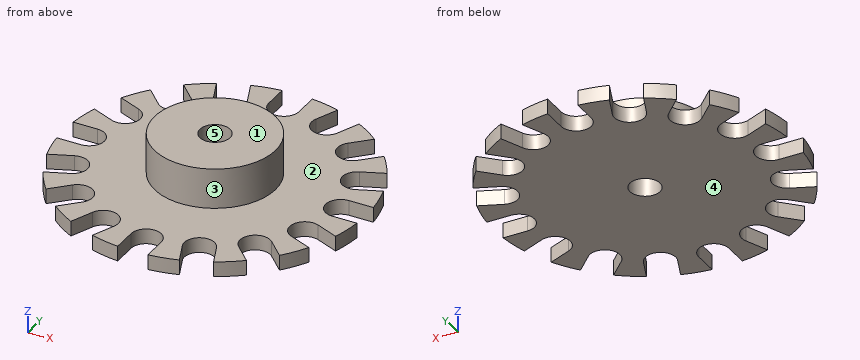
```python
from build123d import *

# Parameters (mm, degrees)
SKETCH1_R           = 15
SKETCH1_R_2         = 1.5
BOSS_EXTRUDE1_DEPTH = 1.5
SKETCH2_R           = 6
SKETCH2_R_2         = 1.5
BOSS_EXTRUDE2_DEPTH = 4
SKETCH3_R           = 1.5
CUT_EXTRUDE3_DEPTH  = 22.587033145


with BuildPart() as part:
    # Sketch1 → Boss-Extrude1 (new body)
    with BuildSketch(Plane.XY):
        Circle(SKETCH1_R)
        Circle(SKETCH1_R_2, mode=Mode.SUBTRACT)
    extrude(amount=BOSS_EXTRUDE1_DEPTH)

    # Sketch2 → Boss-Extrude2 (add)
    with BuildSketch(Plane.XY.offset(1.5)):
        Circle(SKETCH2_R)
        Circle(SKETCH2_R_2, mode=Mode.SUBTRACT)
    extrude(amount=BOSS_EXTRUDE2_DEPTH)

    # Sketch3 → Cut-Extrude3 (cut, through all)
    with BuildSketch(Plane.XY.offset(1.5)):
        with BuildLine():
            ThreePointArc((-1.5, 12.5), (0, 14), (1.5, 12.5))
            Line((1.5, 12.5), (1.5, 14.924811557))
            ThreePointArc((1.5, 14.924811557), (0, 15), (-1.5, 14.924811557))
            Line((-1.5, 14.924811557), (-1.5, 12.5))
        make_face()
        with Locations((0, 12.5)):
            Circle(SKETCH3_R)
        with Locations((4.783542905, 11.548494156)):
            Circle(SKETCH3_R)
        with BuildLine():
            ThreePointArc((7.097297413, 13.214702775), (5.740251485, 13.858192988), (4.325658815, 14.362753072))
            Line((4.325658815, 14.362753072), (3.397723606, 12.122519305))
            ThreePointArc((3.397723606, 12.122519305), (5.076178388, 13.019672077), (6.283542905, 11.548494156))
            ThreePointArc((6.283542905, 11.548494156), (6.254720825, 11.255858673), (6.169362203, 10.974469008))
            Line((6.169362203, 10.974469008), (7.097297413, 13.214702775))
        make_face()
        with Locations((8.838834765, 8.838834765)):
            Circle(SKETCH3_R)
        with BuildLine():
            ThreePointArc((11.614095631, 9.492775288), (10.606601718, 10.606601718), (9.492775288, 11.614095631))
            Line((9.492775288, 11.614095631), (7.778174593, 9.899494937))
            ThreePointArc((7.778174593, 9.899494937), (9.412859913, 10.224654064), (10.338834765, 8.838834765))
            ThreePointArc((10.338834765, 8.838834765), (10.224654064, 8.264809616), (9.899494937, 7.778174593))
            Line((9.899494937, 7.778174593), (11.614095631, 9.492775288))
        make_face()
        with Locations((11.548494156, 4.783542905)):
            Circle(SKETCH3_R)
        with BuildLine():
            ThreePointArc((14.362753072, 4.325658815), (13.858192988, 5.740251485), (13.214702775, 7.097297413))
            Line((13.214702775, 7.097297413), (10.974469008, 6.169362203))
            ThreePointArc((10.974469008, 6.169362203), (12.381849506, 6.030747323), (13.048494156, 4.783542905))
            ThreePointArc((13.048494156, 4.783542905), (12.795698575, 3.950187555), (12.122519305, 3.397723606))
            Line((12.122519305, 3.397723606), (14.362753072, 4.325658815))
        make_face()
        with Locations((12.5, 0)):
            Circle(SKETCH3_R)
        with BuildLine():
            ThreePointArc((15, 0), (14.981191097, 0.750941626), (14.924811557, 1.5))
            Line((14.924811557, 1.5), (12.5, 1.5))
            ThreePointArc((12.5, 1.5), (13.560660172, 1.060660172), (14, 0))
            ThreePointArc((14, 0), (13.560660172, -1.060660172), (12.5, -1.5))
            Line((12.5, -1.5), (14.924811557, -1.5))
            ThreePointArc((14.924811557, -1.5), (14.981191097, -0.750941626), (15, 0))
        make_face()
        with Locations((11.548494156, -4.783542905)):
            Circle(SKETCH3_R)
        with BuildLine():
            ThreePointArc((13.214702775, -7.097297413), (13.858192988, -5.740251485), (14.362753072, -4.325658815))
            Line((14.362753072, -4.325658815), (12.122519305, -3.397723606))
            ThreePointArc((12.122519305, -3.397723606), (12.795698575, -3.950187555), (13.048494156, -4.783542905))
            ThreePointArc((13.048494156, -4.783542905), (12.381849506, -6.030747323), (10.974469008, -6.169362203))
            Line((10.974469008, -6.169362203), (13.214702775, -7.097297413))
        make_face()
        with BuildLine():
            ThreePointArc((9.492775288, -11.614095631), (10.606601718, -10.606601718), (11.614095631, -9.492775288))
            Line((11.614095631, -9.492775288), (9.899494937, -7.778174593))
            ThreePointArc((9.899494937, -7.778174593), (10.224654064, -8.264809616), (10.338834765, -8.838834765))
            ThreePointArc((10.338834765, -8.838834765), (9.412859913, -10.224654064), (7.778174593, -9.899494937))
            Line((7.778174593, -9.899494937), (9.492775288, -11.614095631))
        make_face()
        with Locations((8.838834765, -8.838834765)):
            Circle(SKETCH3_R)
        with Locations((4.783542905, -11.548494156)):
            Circle(SKETCH3_R)
        with BuildLine():
            ThreePointArc((4.325658815, -14.362753072), (5.740251485, -13.858192988), (7.097297413, -13.214702775))
            Line((7.097297413, -13.214702775), (6.169362203, -10.974469008))
            ThreePointArc((6.169362203, -10.974469008), (6.254720825, -11.255858673), (6.283542905, -11.548494156))
            ThreePointArc((6.283542905, -11.548494156), (5.076178388, -13.019672077), (3.397723606, -12.122519305))
            Line((3.397723606, -12.122519305), (4.325658815, -14.362753072))
        make_face()
        with BuildLine():
            ThreePointArc((-1.5, -14.924811557), (0, -15), (1.5, -14.924811557))
            Line((1.5, -14.924811557), (1.5, -12.5))
            ThreePointArc((1.5, -12.5), (0, -14), (-1.5, -12.5))
            Line((-1.5, -12.5), (-1.5, -14.924811557))
        make_face()
        with Locations((0, -12.5)):
            Circle(SKETCH3_R)
        with Locations((-4.783542905, -11.548494156)):
            Circle(SKETCH3_R)
        with BuildLine():
            Line((-6.169362203, -10.974469008), (-7.097297413, -13.214702775))
            ThreePointArc((-7.097297413, -13.214702775), (-5.740251485, -13.858192988), (-4.325658815, -14.362753072))
            Line((-4.325658815, -14.362753072), (-3.397723606, -12.122519305))
            ThreePointArc((-3.397723606, -12.122519305), (-5.357568053, -12.934313455), (-6.169362203, -10.974469008))
        make_face()
        with BuildLine():
            Line((-9.899494937, -7.778174593), (-11.614095631, -9.492775288))
            ThreePointArc((-11.614095631, -9.492775288), (-10.606601718, -10.606601718), (-9.492775288, -11.614095631))
            Line((-9.492775288, -11.614095631), (-7.778174593, -9.899494937))
            ThreePointArc((-7.778174593, -9.899494937), (-9.899494937, -9.899494937), (-9.899494937, -7.778174593))
        make_face()
        with Locations((-8.838834765, -8.838834765)):
            Circle(SKETCH3_R)
        with BuildLine():
            Line((-12.122519305, -3.397723606), (-14.362753072, -4.325658815))
            ThreePointArc((-14.362753072, -4.325658815), (-13.858192988, -5.740251485), (-13.214702775, -7.097297413))
            Line((-13.214702775, -7.097297413), (-10.974469008, -6.169362203))
            ThreePointArc((-10.974469008, -6.169362203), (-12.934313455, -5.357568053), (-12.122519305, -3.397723606))
        make_face()
        with Locations((-11.548494156, -4.783542905)):
            Circle(SKETCH3_R)
        with BuildLine():
            Line((-12.5, 1.5), (-14.924811557, 1.5))
            ThreePointArc((-14.924811557, 1.5), (-15, 0), (-14.924811557, -1.5))
            Line((-14.924811557, -1.5), (-12.5, -1.5))
            ThreePointArc((-12.5, -1.5), (-14, 0), (-12.5, 1.5))
        make_face()
        with Locations((-12.5, 0)):
            Circle(SKETCH3_R)
        with Locations((-11.548494156, 4.783542905)):
            Circle(SKETCH3_R)
        with BuildLine():
            Line((-10.974469008, 6.169362203), (-13.214702775, 7.097297413))
            ThreePointArc((-13.214702775, 7.097297413), (-13.858192988, 5.740251485), (-14.362753072, 4.325658815))
            Line((-14.362753072, 4.325658815), (-12.122519305, 3.397723606))
            ThreePointArc((-12.122519305, 3.397723606), (-12.934313455, 5.357568053), (-10.974469008, 6.169362203))
        make_face()
        with Locations((-8.838834765, 8.838834765)):
            Circle(SKETCH3_R)
        with BuildLine():
            Line((-7.778174593, 9.899494937), (-9.492775288, 11.614095631))
            ThreePointArc((-9.492775288, 11.614095631), (-10.606601718, 10.606601718), (-11.614095631, 9.492775288))
            Line((-11.614095631, 9.492775288), (-9.899494937, 7.778174593))
            ThreePointArc((-9.899494937, 7.778174593), (-9.899494937, 9.899494937), (-7.778174593, 9.899494937))
        make_face()
        with BuildLine():
            Line((-3.397723606, 12.122519305), (-4.325658815, 14.362753072))
            ThreePointArc((-4.325658815, 14.362753072), (-5.740251485, 13.858192988), (-7.097297413, 13.214702775))
            Line((-7.097297413, 13.214702775), (-6.169362203, 10.974469008))
            ThreePointArc((-6.169362203, 10.974469008), (-5.357568053, 12.934313455), (-3.397723606, 12.122519305))
        make_face()
        with Locations((-4.783542905, 11.548494156)):
            Circle(SKETCH3_R)
    extrude(amount=-CUT_EXTRUDE3_DEPTH, mode=Mode.SUBTRACT)


solid = part.part
```
Geometry: final body of the model. Coordinates: model frame, mm. Face numbers are marked on the shaded views. A direction names the side the tool comes from. Coordinates: 2 decimals unless noted, no trailing zeros. Order: outer loops, then holes, each group sorted by start corner. A loop starts at its lowest first (then second) coordinate and runs counter-clockwise, first axis right, second up. Notation, with made-up numbers: (15, -31) -> (43, -31) arc R22 cw to (43, 3) -> close; hole circle Ø8 at (-9, 13). An arc over 180 degrees is marked (long way). Answer in a Markdown table with one row per item.
Item 1: Section D-D on x = 10.5. Output: boundary loops of the cut face in (y, z).
Return value:
| item | result |
|---|---|
| outline | (-8.38, 0) -> (-5.86, 0) -> (-5.86, 1.5) -> (-8.38, 1.5) -> close; (-3.71, 0) -> (3.71, 0) -> (3.71, 1.5) -> (-3.71, 1.5) -> close; (5.86, 0) -> (8.38, 0) -> (8.38, 1.5) -> (5.86, 1.5) -> close |
Item 2: Ray query, L1, parallel to X at y = -3.5, z = 1; L2, parallel to Y at x = 0, z = 2.6; L3, parallel to Z at x = -5.5, y = 5.5. Return the intervals inside material, ascending.
Return value:
| item | result |
|---|---|
| L1 | x = -14.59 to -12.37, -10.77 to 10.77, 12.37 to 14.59 |
| L2 | y = -6 to -1.5, 1.5 to 6 |
| L3 | z = 0 to 1.5 |
Item 3: Contact query for flat-ended pins moving along their axis: P1, Ø0.8, axis at x = 14, z = 1, coming from the +Y side; P2, Ø5, axis at x = -3, y = -8, coming from the +Z side; P3, Ø1.6, axis at y = 13.5, z = 1, coming from the +X side. Output: stop coordinate, or through.
Return value:
| item | result |
|---|---|
| P1 | stops at y = 4.33 |
| P2 | stops at z = 1.5 |
| P3 | stops at x = 7.98 |
Item 4: Draft query along X for the marked faces 3, 4 and 5. Return one class per face: released by +X, released by -X, zero draft, split by the parting line, or undercut.
Return value:
| item | result |
|---|---|
| face 3 | split by the parting line |
| face 4 | zero draft |
| face 5 | undercut |
Item 5: Access query for the marked faces 1 and 2. Directions: +Z, -Z, +X, -X, +Y, -Y. A direction counts if a zero-diameter tool reaches every point of the face in a straight line with its end or side. Return the directions, or none.
Return value:
| item | result |
|---|---|
| face 1 | +Z, +X, -X, +Y, -Y |
| face 2 | +Z |
Item 6: Section C-C on y = -8.5. Output: boundary loops of the cut face in (x, z), plus the area to 3 significant figures.
Return value:
| item | result |
|---|---|
| outline | (-12.36, 0) -> (-10.62, 0) -> (-10.62, 1.5) -> (-12.36, 1.5) -> close; (-7.38, 0) -> (7.38, 0) -> (7.38, 1.5) -> (-7.38, 1.5) -> close; (10.62, 0) -> (12.36, 0) -> (12.36, 1.5) -> (10.62, 1.5) -> close |
| area | 27.3 mm² |
Item 7: Section A-A on y = 0. Output: boundary loops of the cut face in (x, z).
Return value:
| item | result |
|---|---|
| outline | (-11, 0) -> (-1.5, 0) -> (-1.5, 5.5) -> (-6, 5.5) -> (-6, 1.5) -> (-11, 1.5) -> close; (1.5, 0) -> (11, 0) -> (11, 1.5) -> (6, 1.5) -> (6, 5.5) -> (1.5, 5.5) -> close |
